```python
from build123d import *

# Parameters (mm, degrees)
SALIENTE_EXTRUIR1_DEPTH = 2.5
SALIENTE_EXTRUIR2_DEPTH = 7
CROQUIS2_4_R            = 10
SALIENTE_EXTRUIR3_DEPTH = 7.5
REDONDEO1_R             = 4
REDONDEO2_R             = 4
CROQUIS3_R              = 10
SALIENTE_EXTRUIR4_DEPTH = 5
CROQUIS4_R              = 5.05
CORTAR_EXTRUIR1_DEPTH   = 131


with BuildPart() as part:
    # Croquis2 → Saliente-Extruir1 (new, symmetric)
    with BuildSketch(Plane(origin=(0, 0, 0), x_dir=(0, 0, -1), z_dir=(1, 0, 0))):
        with BuildLine():
            ThreePointArc((31.95, 0), (22.592061659, 22.592061659), (0, 31.95))
            Line((0, 31.95), (0, 0))
            Line((0, 0), (31.95, 0))
        make_face()
    extrude(amount=SALIENTE_EXTRUIR1_DEPTH, both=True)

    # Croquis2<3> → Saliente-Extruir2 (add)
    with BuildSketch(Plane(origin=(0, 0, 0), x_dir=(0, 0, -1), z_dir=(1, 0, 0))):
        with BuildLine():
            ThreePointArc((10, 53.9), (7.071067812, 46.828932188), (0, 43.9))
            Line((0, 43.9), (0, 31.95))
            ThreePointArc((0, 31.95), (22.592061659, 22.592061659), (31.95, 0))
            Line((31.95, 0), (43.9, 0))
            ThreePointArc((43.9, 0), (53.9, 10), (63.9, 0))
            ThreePointArc((63.9, 0), (45.184123318, 45.184123318), (0, 63.9))
            ThreePointArc((0, 63.9), (7.071067812, 60.971067812), (10, 53.9))
        make_face()
    extrude(amount=-SALIENTE_EXTRUIR2_DEPTH)

    # Croquis2<4> → Saliente-Extruir3 (add)
    with BuildSketch(Plane(origin=(0, 0, 0), x_dir=(0, 0, -1), z_dir=(1, 0, 0))):
        with Locations((0, 53.9)):
            Circle(CROQUIS2_4_R)
        with Locations((53.9, 0)):
            Circle(CROQUIS2_4_R)
    extrude(amount=-SALIENTE_EXTRUIR3_DEPTH)

    # Redondeo1
    redondeo1_edges = [part.edges().sort_by_distance(p)[0] for p in [
        (0, 0, 0),
    ]]
    fillet(redondeo1_edges, radius=REDONDEO1_R)

    # Redondeo2
    redondeo2_edges = [part.edges().sort_by_distance(p)[0] for p in [
        (-3.5, 43.9, 0),
        (-3.5, 0, -43.9),
    ]]
    fillet(redondeo2_edges, radius=REDONDEO2_R)

    # Croquis3 → Saliente-Extruir4 (add)
    with BuildSketch(Plane(origin=(2.5, 0, 0), x_dir=(0, 0, -1), z_dir=(1, 0, 0))):
        with Locations((4, 4)):
            Circle(CROQUIS3_R)
    extrude(amount=-SALIENTE_EXTRUIR4_DEPTH)

    # Croquis4 → Cortar-Extruir1 (cut)
    with BuildSketch(Plane(origin=(2.5, 0, 0), x_dir=(0, 0, -1), z_dir=(1, 0, 0))):
        with Locations((4, 4)):
            Circle(CROQUIS4_R)
    extrude(amount=-CORTAR_EXTRUIR1_DEPTH, mode=Mode.SUBTRACT)


solid = part.part
```
Input: part model. Units: mm. Frame: model coordinates. A direction names the side the tool comes from. Give positions to 0.01 mm unless a question says otherwise; leave off trailing zeros. Loops run counter-clockwise (first coordinate to the right, second up) from the corner with the lowest first, then second, coordinate; pieces in that order, holes last. Notation, with made-up numbers: (51.25, 78) -> (63.25, 78) arc R23 cw to (63.25, 86) -> close; hole circle Ø10 at (-15, 71). An arc over 180 degrees is marked (long way). Use a Markdown table: item, result.
Q1. Section query D-D, the plane z = -18. Return the cut outline in (x, y).
Entries:
| item | result |
|---|---|
| outline | (-7, 26.4) -> (-2.5, 26.4) -> (-2.5, 0) -> (2.5, 0) -> (2.5, 26.4) -> (0, 26.4) -> (0, 61.31) -> (-7, 61.31) -> close |
Q2. Access query for faces 1 (the flat face through (-2.5, 13, -13)), 2 (the flat face through (0, 27, -26)), 3 (the cylindrical face through (-3.7, -9.76, -51.73)), 4 (the cylindrical face through (-3.549, -0.772, -42.845)), 5 (the flat face through (-1, 27, 0)). Directions: +Z, -Z, +X, -X, +Y, -Y. A direction counts if a zero-diameter tool reaches every point of the face in a straight line with its end or side. Return the directions, or none.
Entries:
| item | result |
|---|---|
| face 1 | +Z, -X, -Y |
| face 2 | -Z, +X, +Y |
| face 3 | -X |
| face 4 | +X, -X, -Y |
| face 5 | +Z, +X, -X |
Q3. Section query C-C, the plane z = -1.5. Return the cut outline in (x, y), plus the area to 3 significant figures.
Entries:
| item | result |
|---|---|
| outline | (-7.5, 44.01) -> (-7, 44.01) -> (-7, 31.91) -> (-2.5, 31.91) -> (-2.5, 8.39) -> (2.5, 8.39) -> (2.5, 31.91) -> (0, 31.91) -> (0, 63.88) -> (-7, 63.88) -> (-7, 63.79) -> (-7.5, 63.79) -> close; (-2.5, -5.68) -> (2.5, -5.68) -> (2.5, -0.39) -> (-2.5, -0.39) -> close |
| area | 378 mm² |
Q4. Ray query, probe 1 along X at (y, z) = (9, -17.5); probe 2 along Y at (x, z) = (0.5, -1); probe 3 along X at (y, z) = (37.5, -15). Return the intervals inside material, ascending. Write a range as from..to.
Entries:
| item | result |
|---|---|
| probe 1 | x = -2.5..2.5 |
| probe 2 | y = -5.54..-0.06, 8.06..31.93 |
| probe 3 | x = -7..0 |
Q5. Section query B-B, the plane y = 4. Return the cut outline in (x, z).
Entries:
| item | result |
|---|---|
| outline | (-7.5, -63.07) -> (-7, -63.07) -> (-7, -63.77) -> (0, -63.77) -> (0, -31.7) -> (2.5, -31.7) -> (2.5, -9.05) -> (-2.5, -9.05) -> (-2.5, -31.7) -> (-7, -31.7) -> (-7, -44.73) -> (-7.5, -44.73) -> close; (-2.5, 1.05) -> (2.5, 1.05) -> (2.5, 6) -> (-2.5, 6) -> close |
Q6. Section query A-A, the plane x = -1. Return the cut outline in (y, z), plus the area to 3 significant figures.
Entries:
| item | result |
|---|---|
| outline | (-2.86, -44.32) arc R10 ccw to (0, -63.9) arc R63.9 ccw to (63.9, 0) arc R10 ccw to (44.32, 2.86) arc R4 cw to (40.48, 0) -> (13.17, 0) arc R10 ccw (long way) to (0, -13.17) -> (0, -40.48) arc R4 cw to start; hole circle Ø10.1 at (4, -4) |
| area | 3,590 mm² |
Q7. Pull-direction query (Y, two-part tool) for faces 6 (the cylindrical face through (-3.549, 42.845, 0.772)), 7 (the cylindrical face through (1.27, 22.34, -22.84)), 8 (the flat face through (-1, 0, -27)), 9 (the flat face through (2.5, 13, -13)); classes: pulls with the +Y half, pulls with the -Y half, needs draft (parallel to the pull), parting line crosses it, or undercut.
Entries:
| item | result |
|---|---|
| face 6 | undercut |
| face 7 | pulls with the +Y half |
| face 8 | pulls with the -Y half |
| face 9 | needs draft |
Q8. First-contact query: P1, Ø1.5, axis at x = -4.5, z = -40.5, coming from the +Y side; P2, Ø3, axis at x = -1.5, z = -33, coming from the -Y side; P3, Ø5, axis at x = -6, z = -23.5, coming from the -Y side. Flat tips, straight axial feed; report the tip coordinate or a pass-through.
Entries:
| item | result |
|---|---|
| P1 | stops at y = 50.03 |
| P2 | stops at y = 0 |
| P3 | stops at y = 18.57 |
